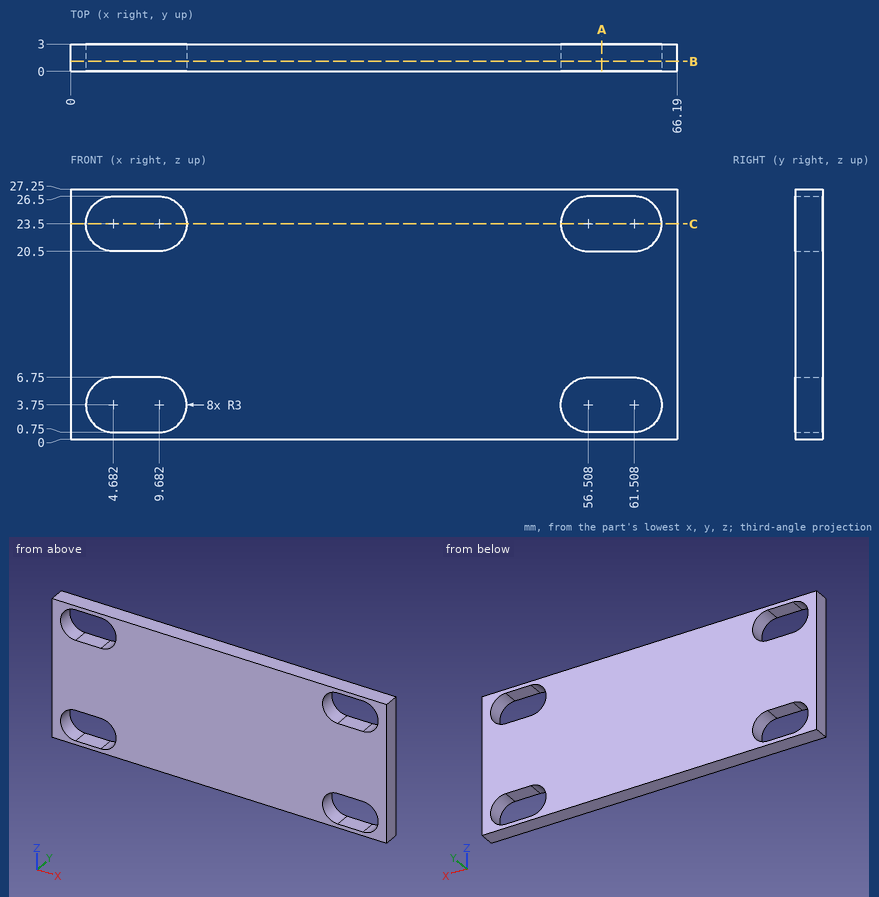
Verification items for this drawing (mm, ordinates from the low corner). Give positions to 0.01 mm unless a question says otherwise; leave off trailing zeros. Loops run counter-clockwise (first coordinate to the right, second up) from the corner with the lowest first, then second, coordinate; pieces in that order, holes last. Notation, with made-up numbers: M -16,-27.75 L 30,-27.75 A23 ccw 30,2.25 Z; hole C 38,56.25 d3. An arc over 180 degrees is marked long. Write item = value, one per line.
(1) Material ranges on line 1 (Z direction, x = 4.5, y = 2.1); line 2 (X direction, y = 2.2, z = 4.25); line 3 (Z direction, x = 55.5, y = 2.35), recorded low to high. Write a range as [from, to].
Answer below:
line_1 = [0, 0.76], [6.74, 20.51], [26.49, 27.25]
line_2 = [0, 1.72], [12.64, 53.55], [64.47, 66.19]
line_3 = [0, 0.92], [6.58, 20.67], [26.33, 27.25]
(2) Sectioned sample at B-B, the plane y = 1.1. Record the cut outline in (x, z).
Answer below:
outline = M 0,0 L 66.19,0 L 66.19,27.25 L 0,27.25 Z; hole M 4.68,0.75 L 9.68,0.75 A3 ccw 9.68,6.75 L 4.68,6.75 A3 ccw Z; hole M 4.68,20.5 L 9.68,20.5 A3 ccw 9.68,26.5 L 4.68,26.5 A3 ccw Z; hole M 56.51,0.75 L 61.51,0.75 A3 ccw 61.51,6.75 L 56.51,6.75 A3 ccw Z; hole M 56.51,20.5 L 61.51,20.5 A3 ccw 61.51,26.5 L 56.51,26.5 A3 ccw Z
(3) Sectioned sample at C-C, the plane z = 23.5. Record the cut outline in (x, y), plus the area to 3 significant figures.
Answer below:
outline = M 0,0 L 1.68,0 L 1.68,3 L 0,3 Z; M 12.68,0 L 53.51,0 L 53.51,3 L 12.68,3 Z; M 64.51,0 L 66.19,0 L 66.19,3 L 64.51,3 Z
area = 133 mm2
(4) Sectioned sample at A-A, the plane x = 58. Record the cut outline in (y, z).
Answer below:
outline = M 0,0 L 3,0 L 3,0.75 L 0,0.75 Z; M 0,6.75 L 3,6.75 L 3,20.5 L 0,20.5 Z; M 0,26.5 L 3,26.5 L 3,27.25 L 0,27.25 Z
